Check sheet for the modelled part. Datum: model origin and axes. Units: mm. Round coordinates to 2 decimals unless told otherwise and drop trailing zeros. Write each loop counter-clockwise with the first axis right and the second up, starting at its lowest first coordinate (ties: lowest second). Pieces come first, ordered by that corner, then holes. Notation, with made-up numbers: M -15,6 L 21,6 A22 cw 21,37 Z; hole C -11,41.25 d2. An arc over 180 degrees is marked long. Put each result on its own line as item: value.
```python
from build123d import *

# Parameters (mm, degrees)
SKETCH_1_R          = 1.65
EXTRUDE_1_DEPTH     = 3
CUT_EXTRUDE_1_DEPTH = 10


with BuildPart() as part:
    # 草图1 → 凸台-拉伸1 (new body)
    with BuildSketch(Plane.XY):
        Polygon((0, 0), (20, 0), (20, -20), (55, -20), (55, 0), (20, 45), (0, 45), align=None)
        with Locations((10, 15)):
            Circle(SKETCH_1_R, mode=Mode.SUBTRACT)
        with Locations((10, 35)):
            Circle(SKETCH_1_R, mode=Mode.SUBTRACT)
        with Locations((10, 25)):
            Circle(SKETCH_1_R, mode=Mode.SUBTRACT)
        with Locations((25, -10)):
            Circle(SKETCH_1_R, mode=Mode.SUBTRACT)
        with Locations((35, -10)):
            Circle(SKETCH_1_R, mode=Mode.SUBTRACT)
        with Locations((45, -10)):
            Circle(SKETCH_1_R, mode=Mode.SUBTRACT)
        with BuildLine():
            Line((20, 10), (20, 28.711779641))
            Line((20, 28.711779641), (42.331384166, 0))
            Line((42.331384166, 0), (30, 0))
            ThreePointArc((30, 0), (22.928932188, 2.928932188), (20, 10))
        make_face(mode=Mode.SUBTRACT)
    extrude(amount=EXTRUDE_1_DEPTH)

    # 草图2 → 切除-拉伸1 (cut)
    with BuildSketch(Plane.XY.offset(3)):
        Polygon((20.5, -19), (61.4403438, -19), (61.4403438, -24.760517067), (16.601724468, -23.670689514), (0, 0), (-5.850932492, 46.668097056), (0.5, 47.42662584), (0.5, 0.5), (20.5, 0.5), align=None)
    extrude(amount=-CUT_EXTRUDE_1_DEPTH, mode=Mode.SUBTRACT)


solid = part.part
```
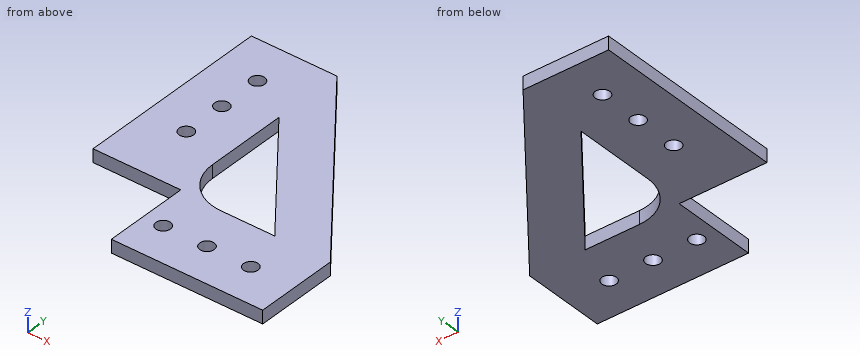
1. Cross-section at B-B (z = 1.15). Enter the section's corners in (x, y), then the cut area to 3 significant figures.
Computed values:
outline: M 0.5,0.5 L 20.5,0.5 L 20.5,-19 L 55,-19 L 55,0 L 20,45 L 0.5,45 Z; hole C 10,15 d3.3; hole C 10,25 d3.3; hole C 10,35 d3.3; hole M 20,10 A10 ccw 30,0 L 42.33,0 L 20,28.71 Z; hole C 25,-10 d3.3; hole C 35,-10 d3.3; hole C 45,-10 d3.3
area: 1,960 mm2
2. Scan lines: probe 1 along Y at (x, z) = (10, 2.35); probe 2 along Y at (x, z) = (25, 1.4); probe 3 along Y at (x, z) = (14.5, 1.6). Record each from-to range of solid material in increasing order.
Computed values:
probe 1: y = 0.5 to 13.35, 16.65 to 23.35, 26.65 to 33.35, 36.65 to 45
probe 2: y = -19 to -11.65, -8.35 to 1.34, 22.28 to 38.57
probe 3: y = 0.5 to 45
3. Cross-section at C-C (x = 10). Enter the section's corners in (y, z), then the cut area to 3 significant figures.
Computed values:
outline: M 0.5,0 L 13.35,0 L 13.35,3 L 0.5,3 Z; M 16.65,0 L 23.35,0 L 23.35,3 L 16.65,3 Z; M 26.65,0 L 33.35,0 L 33.35,3 L 26.65,3 Z; M 36.65,0 L 45,0 L 45,3 L 36.65,3 Z
area: 104 mm2
4. Depth check by flat-ended pin: pin 1 Ø1.5 at (y, z) = (-5.5, 1.5) entering from -X; pin 2 Ø1.5 at (x, z) = (14, 2) entering from -Y; pin 3 Ø1.5 at (y, z) = (16, 2) entering from +X. Enter the tip coordinate at first touch or a pass-through.
Computed values:
pin 1: stops at x = 20.5
pin 2: stops at y = 0.5
pin 3: stops at x = 43.14
5. Cross-section at D-D (y = 25). Enter the section's corners in (x, z), then the cut area to 3 significant figures.
Computed values:
outline: M 0.5,0 L 8.35,0 L 8.35,3 L 0.5,3 Z; M 11.65,0 L 20,0 L 20,3 L 11.65,3 Z; M 22.89,0 L 35.56,0 L 35.56,3 L 22.89,3 Z
area: 86.6 mm2
6. Cross-section at A-A (y = -10). Enter the section's corners in (x, z).
Computed values:
outline: M 20.5,0 L 23.35,0 L 23.35,3 L 20.5,3 Z; M 26.65,0 L 33.35,0 L 33.35,3 L 26.65,3 Z; M 36.65,0 L 43.35,0 L 43.35,3 L 36.65,3 Z; M 46.65,0 L 55,0 L 55,3 L 46.65,3 Z
